Check sheet for the drawn part. Datum: minimum x, y, z corner. Units: mm. A direction names the side the tool comes from. Coordinates: 2 decimals unless noted, no trailing zeros. Write each loop counter-clockwise with the first axis right and the second up, starting at its lowest first coordinate (ties: lowest second). Pieces come first, ordered by that corner, then holes. Notation, with made-up numbers: (25, -1.75) - (43, -1.75) arc R30 cw to (43, 34.25) - close; hole circle Ø5 at (84, -24.5). An arc over 180 degrees is marked (long way). Answer as CSV lines item,"result". Start each with the question number.
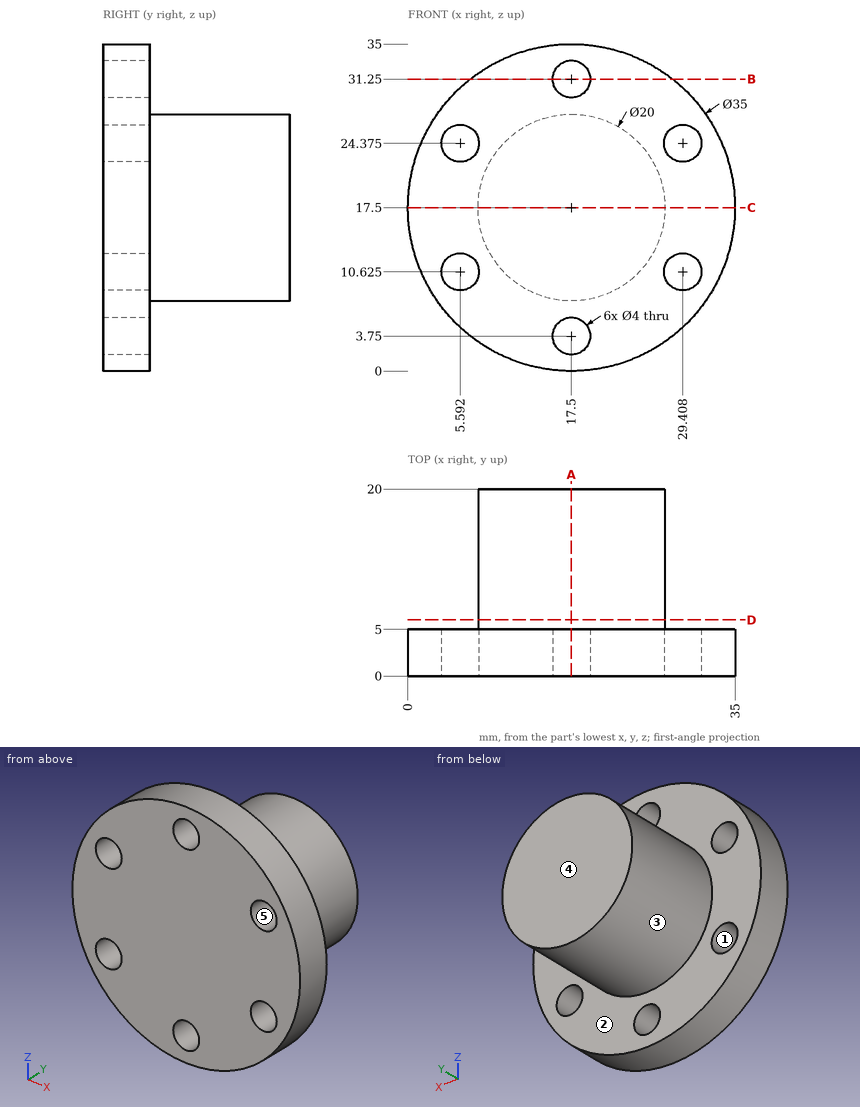
(1) Material ranges on probe 1 along Y at (x, z) = (25.5, 2); probe 2 along X at (y, z) = (12.25, 15.5); probe 3 along Z at (x, y) = (15, 5.5), recorded low to high. Write a range as from..to.
(2) Cross-section at C-C on z = 17.5. Record the boundary of the cut face in (x, y), plus the area to 3 significant figures.
(3) Release check for a two-part mould opening along X. For the marked faces 3, 4 and 5 record: pulls with the +X half, pulls with the -X half, needs draft (parallel to the pull), parting line crosses it, or undercut.
(4) Cross-section at B-B on z = 31.25. Record the boundary of the cut face in (x, y).
(5) Tool access check on the marked faces 1 and 2. Record the directions out of +Z, -Z, +X, -X, +Y, -Y that give a thin tool (end or side, any length) a straight path to the whole face; none if there is none.
(6) Cross-section at D-D on y = 6. Record the boundary of the cut face in (x, z), plus the area to 3 significant figures.
(7) Go/stop test with flat-tipped pins: P1, Ø6, axis at y = 9.5, z = 29, coming from the +X side; P2, Ø10, axis at x = 27.5, z = 29, coming from the +Y side; P3, Ø3, axis at y = 7.5, z = 14, coming from the -X side. Record where each tip stops, or that it passes through.
(8) Cross-section at A-A on x = 17.5. Record the boundary of the cut face in (y, z), plus the area to 3 significant figures.
Checked values:
1,probe 1,"0..5"
1,probe 2,"7.7..27.3"
1,probe 3,"7.82..27.18"
2,outline,"(0, 0) - (35, 0) - (35, 5) - (27.5, 5) - (27.5, 20) - (7.5, 20) - (7.5, 5) - (0, 5) - close"
2,area,"475 mm^2"
3,face 3,"parting line crosses it"
3,face 4,"needs draft"
3,face 5,"undercut"
4,outline,"(6.67, 0) - (15.5, 0) - (15.5, 5) - (6.67, 5) - close; (19.5, 0) - (28.33, 0) - (28.33, 5) - (19.5, 5) - close"
5,face 1,"+Y, -Y"
5,face 2,"+Y"
6,outline,"circle Ø20 at (17.5, 17.5)"
6,area,"314 mm^2"
7,P1,"x = 22.77"
7,P2,"y = 5"
7,P3,"x = 7.7"
8,outline,"(0, 0) - (5, 0) - (5, 1.75) - (0, 1.75) - close; (0, 5.75) - (5, 5.75) - (5, 7.5) - (20, 7.5) - (20, 27.5) - (5, 27.5) - (5, 29.25) - (0, 29.25) - close; (0, 33.25) - (5, 33.25) - (5, 35) - (0, 35) - close"
8,area,"435 mm^2"
